from build123d import *

# Parameters (mm, degrees)
F0_W      = 15
F0_H      = 33
F1_DEPTH  = 3
F2_W      = 15
F2_H      = 2.5
F3_DEPTH  = 2
F4_W      = 15
F4_H      = 5.5
F5_DEPTH  = 1
F7_DEPTH  = 25
F9_DEPTH  = 1.5
F10_W     = 2.5
F10_H     = 21
F11_DEPTH = 1.5
F14_SIZE  = 2.49999
F15_W     = 3
F15_H     = 34.5
F16_DEPTH = 8.25
F17_W     = 8.25
F17_H     = 10
F18_DEPTH = 25
F19_DEPTH = 6
F21_DEPTH = 25
F22_DEPTH = 25


# Not quite as in the source:
# - a fillet or chamfer is up to 0.001 mm smaller than in the source, because OpenCascade refuses the exact size


with BuildPart() as f1:
    # F0 (on Front) → F1 (new body)
    with BuildSketch(Plane.XZ):
        with Locations((7.5, 16.5)):
            Rectangle(F0_W, F0_H)
    extrude(amount=F1_DEPTH)

    # F2 (on face) → F3 (cut)
    with BuildSketch(Plane.XZ.offset(3)):
        with Locations((7.5, 2.25)):
            Rectangle(F2_W, F2_H)
    extrude(amount=-F3_DEPTH, mode=Mode.SUBTRACT)

    # F4 (on face) → F5 (cut)
    with BuildSketch(Plane.XZ.offset(3)):
        with Locations((7.5, 30.25)):
            Rectangle(F4_W, F4_H)
    extrude(amount=-F5_DEPTH, mode=Mode.SUBTRACT)

    # F6 (on face) → F7 (cut)
    with BuildSketch(Plane(origin=(0, 0, 0), x_dir=(-1, 0, 0), z_dir=(0, 1, 0))):
        with BuildLine():
            ThreePointArc((-7.5, 5.9), (-6.5100505063, 6.3100505063), (-6.1, 7.3))
            ThreePointArc((-6.1, 7.3), (-8.4899494937, 8.2899494937), (-7.5, 5.9))
        make_face()
    extrude(amount=-F7_DEPTH, mode=Mode.SUBTRACT)

    # F8 (on face) → F9 (join)
    with BuildSketch(Plane.XY.offset(33)):
        Polygon((16.5, 0), (0, 0), (-1.5, 0), (-1.5, -5), (15, -5), (16.5, -5), align=None)
    extrude(amount=F9_DEPTH)

    # F10 (on face) → F11 (join, through all)
    with BuildSketch(Plane.YZ.offset(16.5)):
        Polygon((0, 34.5), (-5, 34.5), (-5, 21), (-5, 0), (0, 0), align=None)
        with Locations((-6.25, 10.5)):
            Rectangle(F10_W, F10_H)
    extrude(amount=-F11_DEPTH)

    # F13: F1 across plane


with BuildPart() as f1_1:
    add(f1.part)
    add(f1.part.mirror(Plane.YZ.offset(7.5)))

    # F14 (size 2.5 in the source; OpenCascade refuses exactly that, so slightly less here)
    f14_edges = [f1_1.edges().sort_by_distance(p)[0] for p in [
        (15.75, -7.5, 21),
        (-0.75, -7.5, 21),
    ]]
    chamfer(f14_edges, length=F14_SIZE)

    # F15 (on face) → F16 (join)
    with BuildSketch(Plane.YZ.offset(16.5)):
        with Locations((-1.5, 17.25)):
            Rectangle(F15_W, F15_H)
    extrude(amount=F16_DEPTH)

    # F17 (on face) → F18 (cut)
    with BuildSketch(Plane.XZ.offset(3)):
        with Locations((20.625, 29.5)):
            Rectangle(F17_W, F17_H)
    extrude(amount=-F18_DEPTH, mode=Mode.SUBTRACT)

    # F19 (add): a face of the model
    f19_faces = [f1_1.faces().sort_by_distance(p)[0] for p in [
        (20.625, -3, 12.25),
    ]]
    extrude(f19_faces, amount=F19_DEPTH)

    # F20 (on face) → F21 (cut)
    with BuildSketch(Plane(origin=(0, 0, 0), x_dir=(-1, 0, 0), z_dir=(0, 1, 0))):
        with BuildLine():
            ThreePointArc((-22.15, 8.3), (-20.75, 6.9), (-19.35, 8.3))
            Line((-19.35, 8.3), (-20.75, 8.3))
            Line((-20.75, 8.3), (-22.15, 8.3))
        make_face()
        with BuildLine():
            Line((-20.75, 8.3), (-19.35, 8.3))
            ThreePointArc((-19.35, 8.3), (-19.7600505063, 9.2899494937), (-20.75, 9.7))
            Line((-20.75, 9.7), (-20.75, 8.3))
        make_face()
        with BuildLine():
            ThreePointArc((-19.35, 18.3), (-21.7399494937, 19.2899494937), (-20.75, 16.9))
            ThreePointArc((-20.75, 16.9), (-19.7600505063, 17.3100505063), (-19.35, 18.3))
        make_face()
        with BuildLine():
            Line((-22.15, 8.3), (-20.75, 8.3))
            Line((-20.75, 8.3), (-20.75, 9.7))
            ThreePointArc((-20.75, 9.7), (-21.7399494937, 9.2899494937), (-22.15, 8.3))
        make_face()
    extrude(amount=-F21_DEPTH, mode=Mode.SUBTRACT)

    # F22 (cut): a face of the model
    f22_faces = [f1_1.faces().sort_by_distance(p)[0] for p in [
        (20.625, -4.5, 24.5),
    ]]
    extrude(f22_faces, amount=-F22_DEPTH, mode=Mode.SUBTRACT)


solid = f1_1.part
The model under review builds one solid part; all positions refer to its coordinate system, in mm. A direction names the side the tool comes from. Round coordinates to 2 decimals unless told otherwise and drop trailing zeros. Write each loop counter-clockwise with the first axis right and the second up, starting at its lowest first coordinate (ties: lowest second). Pieces come first, ordered by that corner, then holes. Notation, with made-up numbers: (13, 70.5) - (19, 70.5) arc R20 ccw to (19, 74.5) - close; hole circle Ø8 at (47, 85.25). An arc over 180 degrees is marked (long way). One line per item, written item: value. Start each with the question number.
1. To check wall thickness, follow L1, parallel to X at y = -4.25, z = 31; L2, parallel to Z at x = 7.5, y = -0.65; L3, parallel to X at y = -2, z = 7.3. State the ranges of each line that lie inside material, in increasing order. Write a range as from..to.
2. Consider section C-C on y = -4.25. Write out the cut boundary in (x, z).
3. Machinability: for faces 1 (the face through (7, -3, 16)), 2 (the face through (8.1, -5, 33.2)), 3 (the face through (15, -4, 13)), which of the approach directions +Z, -Z, +X, -X, +Y, -Y give a long, thin tool a straight path to every point of the face, cutting with its end or side? Answer none if there is none.
4. Consider section A-A on y = -5.75. Write out the cut boundary in (x, z).
5. Consider section D-D on x = 9.5. Write out the cut boundary in (y, z), and give its area (3 significant figures).
6. Consider section B-B on z = 12.5. Write out the cut boundary in (x, y).
7. The part is to be moulded in two halves that separate along X. For faces 4 (the face through (7, 0, 17)), 5 (the face through (0, -4, 13)), 6 (the face through (7, -2, 1)), 7 (the face through (16.5, -3, 17)), say which applies: released by +X, released by -X, zero draft, split by the parting line, or undercut.
8. Clearance check with flat-ended pins moving along their axes: P1, Ø8, axis at x = 13.5, z = 12, coming from the -Y side; P2, Ø3, axis at x = 7.5, z = 2, coming from the -Y side; P3, Ø0.9, axis at x = 7, y = -3.5, coming from the -Z side; P4, Ø6, axis at x = 2.5, z = 26.5, coming from the -Y side. State where each tip first meets the part, or that it passes through.
Checks:
1. L1: x = -1.5..0, 15..16.5
1. L2: z = 0..5.9, 8.7..34.5
1. L3: x = -1.5..6.1, 8.9..16.5
2. outline: (-1.5, 0) - (0, 0) - (0, 33) - (15, 33) - (15, 0) - (16.5, 0) - (16.5, 34.5) - (-1.5, 34.5) - close
3. face 1: -Z, -Y
3. face 2: +Z, +X, -X, -Y
3. face 3: -Y
4. outline: (-1.5, 0) - (0, 0) - (0, 20.25) - (-1.5, 20.25) - close; (15, 0) - (16.5, 0) - (16.5, 20.25) - (15, 20.25) - close
5. outline: (-5, 33) - (-2, 33) - (-2, 27.5) - (-3, 27.5) - (-3, 3.5) - (-1, 3.5) - (-1, 1) - (-3, 1) - (-3, 0) - (0, 0) - (0, 34.5) - (-5, 34.5) - close
5. area: 96.0 mm^2
6. outline: (-1.5, -7.5) - (0, -7.5) - (0, -3) - (15, -3) - (15, -7.5) - (16.5, -7.5) - (16.5, 0) - (-1.5, 0) - close
7. face 4: zero draft
7. face 5: undercut
7. face 6: undercut
7. face 7: released by +X
8. P1: stops at y = -7.5
8. P2: stops at y = -3
8. P3: stops at z = 33
8. P4: stops at y = -5
